from build123d import *

# Parameters (mm, degrees)
SKETCH1_W           = 63.5
SKETCH1_H           = 233.2736
SKETCH1_R           = 2.413
SKETCH1_R_2         = 4.7625
BOSS_EXTRUDE1_DEPTH = 6.35
CHAMFER1_SIZE       = 2.54


with BuildPart() as part:
    # Sketch1 → Boss-Extrude1 (new body)
    with BuildSketch(Plane.XY):
        with Locations((31.75, 116.6368)):
            Rectangle(SKETCH1_W, SKETCH1_H)
        with Locations((8.382, 215.7476)):
            Circle(SKETCH1_R, mode=Mode.SUBTRACT)
        with Locations((55.118, 215.7476)):
            Circle(SKETCH1_R, mode=Mode.SUBTRACT)
        with Locations((8.382, 169.0116)):
            Circle(SKETCH1_R, mode=Mode.SUBTRACT)
        with Locations((55.118, 169.0116)):
            Circle(SKETCH1_R, mode=Mode.SUBTRACT)
        with Locations((31.75, 192.3796)):
            Circle(SKETCH1_R_2, mode=Mode.SUBTRACT)
    extrude(amount=BOSS_EXTRUDE1_DEPTH)

    # Chamfer1
    chamfer1_edges = [part.edges().sort_by_distance(p)[0] for p in [
        (0, 233.2736, 3.175),
        (63.5, 233.2736, 3.175),
    ]]
    chamfer(chamfer1_edges, length=CHAMFER1_SIZE)


solid = part.part
Source: CAD feature listing. Evaluate the final solid. Frame: model axes, mm. Round coordinates to 2 decimals unless told otherwise and drop trailing zeros. Write each loop counter-clockwise with the first axis right and the second up, starting at its lowest first coordinate (ties: lowest second). Pieces come first, ordered by that corner, then holes. Notation, with made-up numbers: M 12,68.5 L 70,68.5 A23 ccw 70,100.5 Z; hole C 57,-18.75 d5. An arc over 180 degrees is marked long. One line per item, written item: value. Start each with the question number.
Item 1: Pin query (flat end, axial travel): pin 1 (4 mm diameter, centred on x = 8.38, y = 169.01, fed in from +Z). Return the tip coordinate at first contact, or that it passes through.
Item 2: Ray query, L1, parallel to X at y = 193, z = 4.5; L2, parallel to Y at x = 53, z = 4.25; L3, parallel to Y at x = 31.75, z = 3.25. Return the intervals inside material, ascending. Write a range as from..to.
Item 3: Mould query, pull axis X, two halves, no side actions, for faces 1 (the flat face through (31, 233.274, 3)), 2 (the cylindrical face through (7.859, 166.656, 3.131)), 3 (the flat face through (0, 114, 3)). Classes: pulls with the +X half, pulls with the -X half, needs draft (parallel to the pull), parting line crosses it, or undercut.
Item 4: Section query A-A (x = 31.75). Return the cut outline in (y, z), plus the area to 3 significant figures.
Result set:
1. pin 1: passes through
2. L1: x = 0..27.03, 36.47..63.5
2. L2: y = 0..167.86, 170.17..214.59, 216.9..233.27
2. L3: y = 0..187.62, 197.14..233.27
3. face 1: needs draft
3. face 2: undercut
3. face 3: pulls with the -X half
4. outline: M 0,0 L 187.62,0 L 187.62,6.35 L 0,6.35 Z; M 197.14,0 L 233.27,0 L 233.27,6.35 L 197.14,6.35 Z
4. area: 1,420 mm²
